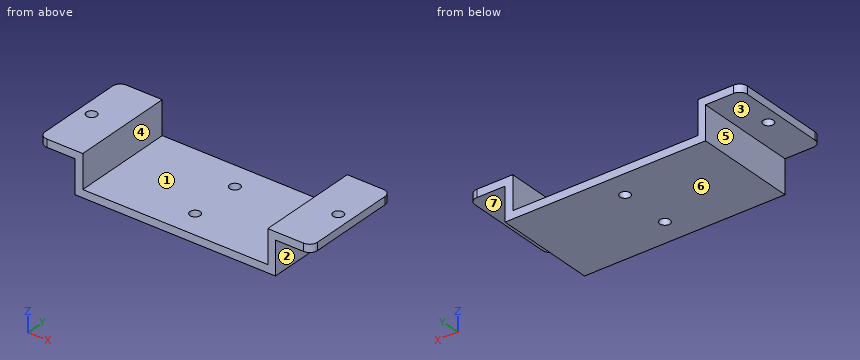
Autodesk Fusion 360 part; units mm, degrees
sketch "Sketch1" plane through (0, 0, 0) normal (0, 0, 1) x (1, 0, 0)
  line L0 (0, 0) -> (78, 0)
  line L1 (78, 0) -> (78, 40)
  line L2 (78, 40) -> (0, 40)
  line L3 (0, 40) -> (0, 0)
  dimension "d1" = 78
  dimension "d2" = 40
extrude "Extrude1" add sketch "Sketch1" along normal blind 3
sketch "Sketch3" plane through (0, 0, 3) normal (0, 0, 1) x (-1, 0, 0)
  line L0 (0, -40) -> (0, 0)
  line L1 (0, 0) -> (-78, 0)
  line L2 (-78, 0) -> (-78, -40)
  line L3 (-78, -40) -> (0, -40)
  line L4 (0, -40) -> (-3, -40)
  line L5 (-3, -40) -> (-3, 0)
  line L6 (0, 0) -> (0, -40)
  dimension "d5" = 3
extrude "Extrude2" add sketch "Sketch3" along normal blind 13 contours L0 L1 L3 L4 L5 L6
sketch "Sketch4" plane through (0, 0, 3) normal (0, 0, 1) x (-1, 0, 0)
  line L0 (-3, -40) -> (-3, 0)
  line L1 (-3, 0) -> (-78, 0)
  line L2 (-78, 0) -> (-78, -40)
  line L3 (-78, -40) -> (-3, -40)
  line L4 (-78, -40) -> (-75, -40)
  line L5 (-75, -40) -> (-75, 0)
  line L6 (-78, 0) -> (-78, -40)
  dimension "d8" = 3
extrude "Extrude3" add sketch "Sketch4" along normal blind 13 contours L1 L2 L3 L4 L5 L6
sketch "Sketch5" plane through (78, 0, 0) normal (1, 0, 0) x (0, 1, 0)
  line L0 (0, 0) -> (40, 0)
  line L1 (40, 0) -> (40, 16)
  line L2 (40, 16) -> (0, 16)
  line L3 (0, 16) -> (0, 0)
  line L4 (40, 16) -> (40, 13)
  line L5 (40, 13) -> (0, 13)
  line L6 (0, 13) -> (0, 16)
extrude "Extrude4" add sketch "Sketch5" along normal blind 14 contours L1 L2 L3 L4 L5 L6
sketch "Sketch6" plane through (0, 0, 0) normal (-1, 0, 0) x (0, -1, 0)
  line L0 (-40, 0) -> (0, 0)
  line L1 (0, 0) -> (0, 16)
  line L2 (0, 16) -> (-40, 16)
  line L3 (-40, 16) -> (-40, 0)
  line L4 (-40, 16) -> (0, 16)
  line L5 (0, 16) -> (0, 13)
  line L6 (0, 13) -> (-40, 13)
  line L7 (-40, 13) -> (-40, 16)
extrude "Extrude5" add sketch "Sketch6" along normal blind 14 contours L1 L2 L3 L4 L5 L6 L7
sketch "Sketch7" plane through (0, 0, 16) normal (0, 0, 1) x (-1, 0, 0)
  line L0 (14, 0) -> (-3, 0)
  line L1 (-3, 0) -> (-3, -40)
  line L2 (-3, -40) -> (14, -40)
  line L3 (14, -40) -> (14, 0)
  circle A0 centre (9, -20) radius 2
  dimension "d15" = 4
extrude "Extrude6" cut sketch "Sketch7" against normal blind 3 contours A0
sketch "Sketch8" plane through (0, 0, 16) normal (0, 0, 1) x (-1, 0, 0)
  line L0 (-92, -40) -> (-75, -40)
  line L1 (-75, -40) -> (-75, 0)
  line L2 (-75, 0) -> (-92, 0)
  line L3 (-92, 0) -> (-92, -40)
  line L4 (-92, -20) -> (-87, -20)
  circle A0 centre (-87, -20) radius 2
  dimension "d18" = 4
extrude "Extrude7" cut sketch "Sketch8" against normal blind 3 contours A0
fillet "Fillet1" radius 3 1 edges at (-14, 0, 14.5)
fillet "Fillet2" radius 3 1 edges at (-14, 40, 14.5)
fillet "Fillet3" radius 3 1 edges at (92, 0, 14.5)
fillet "Fillet4" radius 3 1 edges at (92, 40, 14.5)
sketch "Sketch9" plane through (0, 0, 3) normal (0, 0, 1) x (-1, 0, 0)
  line L0 (-75, 0) -> (-75, -40)
  line L1 (-75, -40) -> (-3, -40)
  line L2 (-3, -40) -> (-3, 0)
  line L3 (-3, 0) -> (-75, 0)
  line L4 (-39, -40) -> (-39, 0)
  line L5 (-3, -20) -> (-75, -20)
  circle A0 centre (-39, -30) radius 2
  circle A1 centre (-39, -10) radius 2
  dimension "d25" = 4
  dimension "d26" = 4
  dimension "d27" = 10
  dimension "d28" = 10
extrude "Extrude8" cut sketch "Sketch9" against normal blind 3 contours L4 A1 | L4 A1 | L4 A0 | L4 A0
Verification items for the finished model (mm, model axes). Face numbers are marked on the shaded views. A direction names the side the tool comes from. Coordinates: 2 decimals unless noted, no trailing zeros. Write each loop counter-clockwise with the first axis right and the second up, starting at its lowest first coordinate (ties: lowest second). Pieces come first, ordered by that corner, then holes. Notation, with made-up numbers: M 24.5,21.5 L 38.5,21.5 A32 ccw 38.5,58.5 Z; hole C -37.75,9 d7. An arc over 180 degrees is marked long. Use a Markdown table: item, result.
Q1. Go/stop test with flat-tipped pins: P1, Ø2.5, axis at x = 39, y = 30, coming from the -Z side; P2, Ø4, axis at y = 18, z = 7, coming from the -X side; P3, Ø11, axis at x = -7, y = 18.5, coming from the -Z side; P4, Ø6.5, axis at y = 16, z = 8.5, coming from the +X side. Record where each tip stops, or that it passes through.
Reply:
| item | result |
|---|---|
| P1 | passes through |
| P2 | stops at x = 0 |
| P3 | stops at z = 13 |
| P4 | stops at x = 78 |
Q2. Sectioned sample at C-C, the plane y = 10. Record the boundary of the cut face in (x, z).
Reply:
| item | result |
|---|---|
| outline | M -14,13 L 0,13 L 0,0 L 37,0 L 37,3 L 3,3 L 3,16 L -14,16 Z; M 41,0 L 78,0 L 78,13 L 92,13 L 92,16 L 75,16 L 75,3 L 41,3 Z |
Q3. Thickness scan on line 1 (X direction, y = 20, z = 15); line 2 (Y direction, x = 39, z = 0.95); line 3 (X direction, y = 10, z = 1.5). Record the ranges inside material, lowest first.
Reply:
| item | result |
|---|---|
| line 1 | x = -14 to -11, -7 to 3, 75 to 85, 89 to 92 |
| line 2 | y = 0 to 8, 12 to 28, 32 to 40 |
| line 3 | x = 0 to 37, 41 to 78 |
Q4. Sectioned sample at A-A, the plane x = -9. Record the boundary of the cut face in (y, z), plus the area to 3 significant figures.
Reply:
| item | result |
|---|---|
| outline | M 0,13 L 18,13 L 18,16 L 0,16 Z; M 22,13 L 40,13 L 40,16 L 22,16 Z |
| area | 108 mm² |
Q5. Set-up check for the marked faces 4, 5, 6 and 7: record each of +Z, -Z, +X, -X, +Y, -Y from which the full face is reachable in a straight line by a thin tool's end or side.
Reply:
| item | result |
|---|---|
| face 4 | +Z, +Y, -Y |
| face 5 | -Z, -X, +Y, -Y |
| face 6 | -Z, +X, -X, +Y, -Y |
| face 7 | -Z, +X, +Y, -Y |
Q6. Draft check along X on the marked faces 1, 2 and 3. Enter one of: +X half, -X half, draft (parallel to the pull), parting line (faces both ways), or undercut.
Reply:
| item | result |
|---|---|
| face 1 | undercut |
| face 2 | +X half |
| face 3 | draft |
Q7. Sectioned sample at B-B, the plane y = 20. Record the boundary of the cut face in (x, z), plus the area to 3 significant figures.
Reply:
| item | result |
|---|---|
| outline | M -14,13 L -11,13 L -11,16 L -14,16 Z; M -7,13 L 0,13 L 0,0 L 78,0 L 78,13 L 85,13 L 85,16 L 75,16 L 75,3 L 3,3 L 3,16 L -7,16 Z; M 89,13 L 92,13 L 92,16 L 89,16 Z |
| area | 372 mm² |
Q8. Sectioned sample at D-D, the plane x = 39. Record the boundary of the cut face in (y, z).
Reply:
| item | result |
|---|---|
| outline | M 0,0 L 8,0 L 8,3 L 0,3 Z; M 12,0 L 28,0 L 28,3 L 12,3 Z; M 32,0 L 40,0 L 40,3 L 32,3 Z |
